from build123d import *

# Parameters (mm, degrees)
ESQUISSE1_W             = 47
ESQUISSE1_H             = 31.9
BOSS_EXTRU_1_DEPTH      = 1.5
ESQUISSE2_W             = 2.5
ESQUISSE2_H             = 4.7
ENL_V_MAT_EXTRU_1_DEPTH = 2.5
ESQUISSE3_R             = 2.5
ESQUISSE3_W             = 6
ESQUISSE3_H             = 4
BOSS_EXTRU_2_DEPTH      = 6.599064
ESQUISSE4_W             = 3
ESQUISSE4_H             = 4
BOSS_EXTRU_3_DEPTH      = 3
ESQUISSE4_3_R           = 0.75
ENL_V_MAT_EXTRU_2_DEPTH = 5


with BuildPart() as part:
    # Esquisse1 → Boss.-Extru.1 (new body)
    with BuildSketch(Plane.XY):
        with Locations((23.5, 15.95)):
            Rectangle(ESQUISSE1_W, ESQUISSE1_H)
    extrude(amount=BOSS_EXTRU_1_DEPTH)

    # Esquisse2 → Enl_v. mat.-Extru.1 (cut, through all)
    with BuildSketch(Plane.XY.offset(1.5)):
        with Locations((45.75, 29.55)):
            Rectangle(ESQUISSE2_W, ESQUISSE2_H)
        with Locations((45.75, 2.35)):
            Rectangle(ESQUISSE2_W, ESQUISSE2_H)
        with Locations((1.25, 2.35)):
            Rectangle(ESQUISSE2_W, ESQUISSE2_H)
        with Locations((1.25, 29.55)):
            Rectangle(ESQUISSE2_W, ESQUISSE2_H)
    extrude(amount=-ENL_V_MAT_EXTRU_1_DEPTH, mode=Mode.SUBTRACT)

    # Esquisse3 → Boss.-Extru.2 (add)
    with BuildSketch(Plane.XY.offset(1.5)):
        with Locations((39.474011, 29.2125)):
            Circle(ESQUISSE3_R)
        with Locations((39.474011, 13.6925)):
            Circle(ESQUISSE3_R)
        with Locations((9.014011, 29.2125)):
            Rectangle(ESQUISSE3_W, ESQUISSE3_H)
        with Locations((9.014011, 13.6925)):
            Rectangle(ESQUISSE3_W, ESQUISSE3_H)
    extrude(amount=BOSS_EXTRU_2_DEPTH)

    # Esquisse4 → Boss.-Extru.3 (add)
    with BuildSketch(Plane.XY.offset(8.099064)):
        with Locations((7.514011, 13.6925)):
            Rectangle(ESQUISSE4_W, ESQUISSE4_H)
        with Locations((7.514011, 29.2125)):
            Rectangle(ESQUISSE4_W, ESQUISSE4_H)
    extrude(amount=BOSS_EXTRU_3_DEPTH)

    # Esquisse4_3 → Enl_v. mat.-Extru.2 (cut)
    with BuildSketch(Plane.XY.offset(8.099064)):
        with Locations((39.474011, 29.2125)):
            Circle(ESQUISSE4_3_R)
        with Locations((39.474011, 13.6925)):
            Circle(ESQUISSE4_3_R)
    extrude(amount=-ENL_V_MAT_EXTRU_2_DEPTH, mode=Mode.SUBTRACT)


solid = part.part
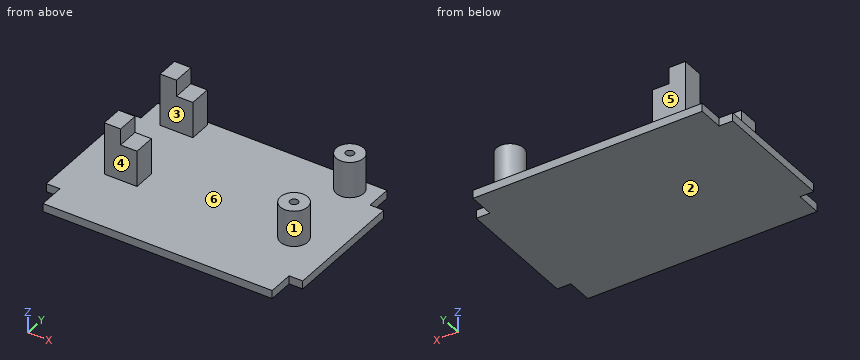
Part model, mm, in its own coordinate system. Face numbers are marked on the shaded views. A direction names the side the tool comes from. Coordinates: 2 decimals unless noted, no trailing zeros. Loops run counter-clockwise (first coordinate to the right, second up) from the corner with the lowest first, then second, coordinate; pieces in that order, holes last. Notation, with made-up numbers: (-37.5, 61) -> (-29.5, 61) arc R13 cw to (-29.5, 78) -> close; hole circle Ø1 at (-36.75, 47). An arc over 180 degrees is marked (long way). Use a Markdown table: item, result. Add a question column.
Item 1: Band-saw the part on A-A on z = 9. Write the cut outline in (x, y), plus the area to 3 significant figures.
Item 2: Which spindle directions (+Z, -Z, +X, -X, +Y, -Y) get a long thin tool onto all of the face, cutting with end or side? Do the marked faces 1, 2, 3 and 4. Say none if no direction does.
Item 3: Band-saw the part on B-B on z = 5.5. Write the cut outline in (x, y), plus the area to 3 significant figures.
Item 4: Flat gauge pins, fed straight in: P1, Ø1.5, axis at x = 11.5, z = 8.5, coming from the -Y side; P2, Ø1.5, axis at x = 11, y = 28.5, coming from the +Z side; P3, Ø5, axis at y = 15.5, z = 9, coming from the -X side; P4, Ø2, axis at x = 15, z = 5.5, coming from the -Y side. Where does each tip first touch, or does it go through?
Item 5: Pull direction X, two halves, no side cores. Call the marked faces 5 and 6: +X half, -X half, draft (parallel to the pull), parting line (faces both ways), or undercut.
Item 6: Band-saw the part on D-D on x = 31. Write the cut outline in (y, z).
Item 7: Probe probe 1 along Y at (x, z) = (37.5, 2.5); probe 2 along Z at (x, y) = (44, 25); probe 3 along X at (y, z) = (12, 6.75). List the from-to ranges inside material, lowest first.
Item 8: Band-saw the part on C-C on y = 30.5. Write the cut outline in (x, z), plus the area to 3 significant figures.
Geometry says:
| question | item | result |
|---|---|---|
| 1 | outline | (6.01, 11.69) -> (9.01, 11.69) -> (9.01, 15.69) -> (6.01, 15.69) -> close; (6.01, 27.21) -> (9.01, 27.21) -> (9.01, 31.21) -> (6.01, 31.21) -> close |
| 1 | area | 24.0 mm² |
| 2 | face 1 | +Z |
| 2 | face 2 | -Z, +X, -X, +Y, -Y |
| 2 | face 3 | +Z, -X |
| 2 | face 4 | +Z, -X, -Y |
| 3 | outline | (6.01, 11.69) -> (12.01, 11.69) -> (12.01, 15.69) -> (6.01, 15.69) -> close; (6.01, 27.21) -> (12.01, 27.21) -> (12.01, 31.21) -> (6.01, 31.21) -> close; circle Ø5 at (39.47, 13.69); circle Ø5 at (39.47, 29.21); hole circle Ø1.5 at (39.47, 13.69); hole circle Ø1.5 at (39.47, 29.21) |
| 3 | area | 83.7 mm² |
| 4 | P1 | y = 11.69 |
| 4 | P2 | z = 8.1 |
| 4 | P3 | x = 6.01 |
| 4 | P4 | through |
| 5 | face 5 | draft |
| 5 | face 6 | undercut |
| 6 | outline | (0, 0) -> (31.9, 0) -> (31.9, 1.5) -> (0, 1.5) -> close |
| 7 | probe 1 | 12.16 to 15.23, 27.68 to 30.75 |
| 7 | probe 2 | 0 to 1.5 |
| 7 | probe 3 | 6.01 to 12.01, 37.63 to 41.31 |
| 8 | outline | (2.5, 0) -> (44.5, 0) -> (44.5, 1.5) -> (41.62, 1.5) -> (41.62, 8.1) -> (37.33, 8.1) -> (37.33, 1.5) -> (12.01, 1.5) -> (12.01, 8.1) -> (9.01, 8.1) -> (9.01, 11.1) -> (6.01, 11.1) -> (6.01, 1.5) -> (2.5, 1.5) -> close |
| 8 | area | 140 mm² |
